Could you check a few things on this model? Use its own coordinates, in mm. Face numbers are marked on the shaded views. A direction names the side the tool comes from. Give positions to 0.01 mm unless a question says otherwise; leave off trailing zeros. Write each loop counter-clockwise with the first axis right and the second up, starting at its lowest first coordinate (ties: lowest second). Pieces come first, ordered by that corner, then holes. Notation, with made-up numbers: (12, -36) - (71, -36) arc R33 ccw to (71, -8) - close; hole circle Ø6 at (-11, 21.5). An arc over 180 degrees is marked (long way). Answer as a JSON object with one key per item and string values. Group by question number.
```python
from build123d import *

# Parameters (mm, degrees)
F0_R     = 5
F1_DEPTH = 5
F2_R     = 1.5
F4_DEPTH = 20
F3_R     = 7.5
F3_R_2   = 4.5
F5_DEPTH = 2


with BuildPart() as f1:
    # F0 (on Top) → F1 (new body)
    with BuildSketch(Plane.XY):
        Circle(F0_R)
    extrude(amount=F1_DEPTH)

    # F2 (on face) → F4 (join)
    with BuildSketch(Plane.XY.offset(5)):
        Circle(F2_R)
    extrude(amount=F4_DEPTH)

    # F3 (on Front) → F5 (join, symmetric)
    with BuildSketch(Plane.XZ):
        with Locations((0, 29.75847)):
            Circle(F3_R)
        with Locations((0, 29.75847)):
            Circle(F3_R_2, mode=Mode.SUBTRACT)
    extrude(amount=F5_DEPTH, both=True)

    # F3 (on Front) → F6 (revolve)
    with BuildSketch(Plane.XZ):
        Polygon((5, 5), (0, 12.11049), (0, 5), align=None)
    revolve(axis=Axis((0, 0, 8.555245), (0, 0, -1)))


solid = f1.part
```
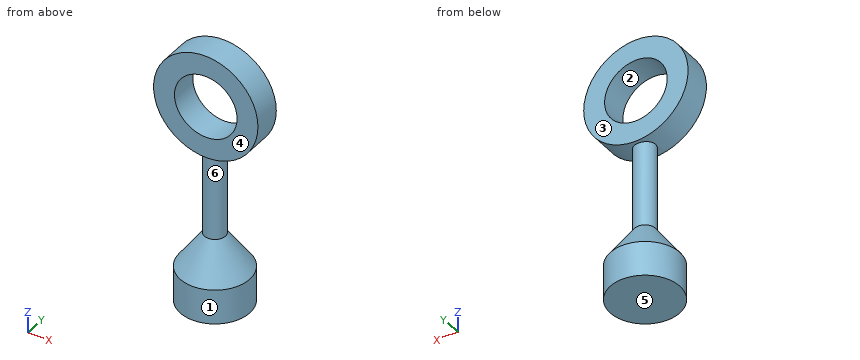
(1) For the marked faces 4, 5 and 6, which set-ups out of +Z, -Z, +X, -X, +Y, -Y let a thin tool reach every point of the face, with its end or its side?
(2) I want a section at B-B, the plane z = 26.5. Please give me the cut outline in (x, y).
(3) I want a section at A-A, the plane x = 0. Please give me the cut outline in (y, z).
(4) If we mould it in two halves opening along X, with no side actions, what happens to the marked faces 1, 2 and 3? For each: +X half, -X half, draft (parallel to the pull), parting line (faces both ways), or undercut.
(5) I want a section at C-C, the plane y = 0. Please give me the cut outline in (x, z), and give its area (3 significant figures).
(6) Will these pins go through, and if not, where does the flat tip stop? P1, Ø2, axis at y = 2, z = 11.5, coming from the -X side; P2, Ø8, axis at x = 3.5, z = 19, coming from the +Y side; P3, Ø3, axis at x = -3, y = -1.5, coming from the +Z side.
(7) I need wall thicknesses on L1, parallel to Z at x = 3, y = 0.5; L2, parallel to Z at x = 0, y = 0.35; L3, parallel to X at y = 0.25, z = 3. Which ranges of each line are inside material? Lowest first, please.
(8) I want a section at D-D, the plane z = 3. Please give me the cut outline in (x, y).
Entries:
{
 "1": {"face 4": "+Z, +X, -X, -Y", "face 5": "-Z, +X, -X, +Y, -Y", "face 6": "none"},
 "2": {"outline": "(-6.76, -2) - (-3.1, -2) - (-3.1, 2) - (-6.76, 2) - close; (3.1, -2) - (6.76, -2) - (6.76, 2) - (3.1, 2) - close"},
 "3": {"outline": "(-5, 0) - (5, 0) - (5, 5) - (1.5, 9.98) - (1.5, 22.26) - (2, 22.26) - (2, 25.26) - (-2, 25.26) - (-2, 22.26) - (-1.5, 22.26) - (-1.5, 9.98) - (-5, 5) - close; (-2, 34.26) - (2, 34.26) - (2, 37.26) - (-2, 37.26) - close"},
 "4": {"face 1": "parting line", "face 2": "undercut", "face 3": "draft"},
 "5": {"outline": "(-5, 0) - (5, 0) - (5, 5) - (1.5, 9.98) - (1.5, 22.41) arc R7.5 ccw (long way) to (-1.5, 22.41) - (-1.5, 9.98) - (-5, 5) - close; hole circle Ø9 at (0, 29.76)", "area": "232 mm^2"},
 "6": {"P1": "x = -1.12", "P2": "y = 2", "P3": "z = 37.11"},
 "7": {"L1": "0 to 7.79, 22.88 to 26.4, 33.11 to 36.63", "L2": "0 to 25.26, 34.26 to 37.26", "L3": "-4.99 to 4.99"},
 "8": {"outline": "circle Ø10 at (0, 0)"}
}
